Autodesk Inventor part; units mm, degrees
ref_plane "YZ Plane" through (0, 0, 0) normal (1, 0, 0) x (0, 1, 0)
ref_plane "XZ Plane" through (0, 0, 0) normal (0, 1, 0) x (-1, 0, 0)
ref_plane "XY Plane" through (0, 0, 0) normal (0, 0, 1) x (1, 0, 0)
sketch "Sketch1" plane through (0, 0, 0) normal (0, 0, 1) x (1, 0, 0)
  line L0 (-35, -5) -> (35, -5)
  line L1 (35, -5) -> (35, 5)
  line L2 (35, 5) -> (-35, 5)
  line L3 (-35, 5) -> (-35, -5)
  line L4 (-35, -5) -> (35, 5) construction
  line L5 (35, -5) -> (-35, 5) construction
  point P0 (0, 0)
  dimension "d0" = 70
  dimension "d1" = 10
extrude "Extrusion1" add sketch "Sketch1" along normal blind 1
sketch "Sketch2" plane through (0, 0, 1) normal (0, 0, 1) x (1, 0, 0)
  line L0 (-30.5, 0) -> (30.5, 0) construction
  point P0 (0, 0)
  point P1 (0, 0)
  dimension "d4" = 61
hole "Hole1" at (-30.5, 0, 1) at (30.5, 0, 1) direction (0, 0, -1) diameter 6.6 depth 8 tip angle 118
properties part number "Cap_CU_Oben" material "Copper"
Check sheet for the modelled part. Datum: model origin and axes. Units: mm. Give positions to 0.01 mm unless a question says otherwise; leave off trailing zeros. Write each loop counter-clockwise with the first axis right and the second up, starting at its lowest first coordinate (ties: lowest second). Pieces come first, ordered by that corner, then holes.
Item 1: Draft check along Y on faces 1 (the face through (0, 0, 0)), 2 (the face through (-33.283, -1.774, 0.493)). Enter one of: released by +Y, released by -Y, zero draft, split by the parting line, or undercut.
Item 2: Cross-section at C-C (z = 0.6). Enter the section's corners in (x, y).
Item 3: Cross-section at B-B (y = 0). Enter the section's corners in (x, z), and give its area (3 significant figures).
Item 4: Scan lines: L1, parallel to X at y = 0, z = 0.45; L2, parallel to Y at x = -30.5, z = 0.6; L3, parallel to X at y = -1.75, z = 0.95. Record each from-to range of solid material in increasing order.
Item 5: Cross-section at A-A (x = -30.5). Enter the section's corners in (y, z), and give its area (3 significant figures).
Item 6: Gauge pin test, flat end, axial feed: pin 1 (2 mm diameter, centred on x = -6, y = 2, fed in from -Z). Record the tip position at first contact, or that the pin passes through.
Report:
1. face 1: zero draft
1. face 2: undercut
2. outline: (-35, -5) - (35, -5) - (35, 5) - (-35, 5) - close; hole circle Ø6.6 at (-30.5, 0); hole circle Ø6.6 at (30.5, 0)
3. outline: (-35, 0) - (-33.8, 0) - (-33.8, 1) - (-35, 1) - close; (-27.2, 0) - (27.2, 0) - (27.2, 1) - (-27.2, 1) - close; (33.8, 0) - (35, 0) - (35, 1) - (33.8, 1) - close
3. area: 56.8 mm2
4. L1: x = -35 to -33.8, -27.2 to 27.2, 33.8 to 35
4. L2: y = -5 to -3.3, 3.3 to 5
4. L3: x = -35 to -33.3, -27.7 to 27.7, 33.3 to 35
5. outline: (-5, 0) - (-3.3, 0) - (-3.3, 1) - (-5, 1) - close; (3.3, 0) - (5, 0) - (5, 1) - (3.3, 1) - close
5. area: 3.40 mm2
6. pin 1: stops at z = 0
